Work out the finished part from the listing and answer in its coordinate system (mm). A direction names the side the tool comes from. Coordinates: 2 decimals unless noted, no trailing zeros. Order: outer loops, then holes, each group sorted by start corner. A loop starts at its lowest first (then second) coordinate and runs counter-clockwise, first axis right, second up. Notation, with made-up numbers: M 60,-0.5 L 107,-0.5 A15 ccw 107,19.5 Z; hole C 31.25,-14 d11. An arc over 180 degrees is marked long. Use a Markdown table: item, result. Add a question column.
from build123d import *

# Parameters (mm, degrees)
SKETCH_W        = 3.5
SKETCH_H        = 15
PAD_DEPTH       = 4
SKETCH001_R     = 1.65
PAD001_DEPTH    = 6
POCKET_DEPTH    = 3
POCKET001_DEPTH = 15.001


with BuildPart() as part:
    # Sketch → Pad (new body)
    with BuildSketch(Plane.XY):
        with Locations((1.75, 7.5)):
            Rectangle(SKETCH_W, SKETCH_H)
    extrude(amount=PAD_DEPTH)

    # Sketch001 → Pad001 (join)
    with BuildSketch(Plane.XY):
        with Locations((1.75, 2.5)):
            Circle(SKETCH001_R)
    extrude(amount=PAD001_DEPTH)

    # Sketch002 (on Face1 of Pad001) → Pocket (cut)
    with BuildSketch(Plane.XZ):
        Polygon((3.25, 3.75), (3.25, 0.25), (0.25, 0.25), (0.25, 3.75), (1.75, 3.75), align=None)
    extrude(amount=-POCKET_DEPTH, mode=Mode.SUBTRACT)

    # Sketch003 → Pocket001 (cut, through all)
    with BuildSketch(Plane.XZ):
        Polygon((0.75, 3.75), (1.75, 3.75), (2.75, 3.75), (2.75, 2.25), (0.75, 2.25), align=None)
    extrude(amount=-POCKET001_DEPTH, mode=Mode.SUBTRACT)


solid = part.part
(1) A cutting plane is placed at B-B on x = 1.75. Write down the section's boundary in (y, z).
(2) Straight lines are drawn through the part: line 1 (Z direction, x = 2.1, y = 1.25); line 2 (Z direction, x = 2.1, y = 13); line 3 (X direction, y = 8, z = 2.5). For each, find the intervals that lie inside material, in ascending order.
(3) A cutting plane is placed at A-A on z = 3.2. Write down the section's boundary in (x, y), plus the area to 3 significant figures.
(4) A cutting plane is placed at C-C on y = 11.5. Write down the section's boundary in (x, z), plus the area to 3 significant figures.
(5) Which of the six approach directions +Z, -Z, +X, -X, +Y, -Y give full straight-line access (tool end or side, diameter ignored) to faces 1 (the cylindrical face through (2.64, 3.89, 4.99)), 2 (the flat face through (3.25, 1, 2)), 3 (the flat face through (2.75, 9, 3)), 4 (the flat face through (2, 3, 6)), 5 (the flat face through (2, 15, 2))?
(6) Given P1, Ø1.6, axis at x = 2, y = 7, coming from the +Z side; P2, Ø1.5, axis at x = 1.5, y = 8, coming from the -Z side; P3, Ø1.5, axis at y = 3.5, z = 5.5, coming from the +X side, each flat-ended and moving along its own axis, determine where each tip first touches the part or whether it passes through.
(7) A cutting plane is placed at D-D on z = 1.15. Write down the section's boundary in (x, y).
(8) The mould has two halves that part along Z. Classify faces 6 (the flat face through (2, 9, 2.25)), 7 (the flat face through (2, 9, 4)), 8 (the flat face through (3.5, 7, 2)): pulls with the +Z half, pulls with the -Z half, needs draft (parallel to the pull), parting line crosses it, or undercut.
From the geometry:
| question | item | result |
|---|---|---|
| 1 | outline | M 0,0 L 15,0 L 15,2.25 L 3,2.25 L 3,0.25 L 0,0.25 Z; M 0,3.75 L 15,3.75 L 15,4 L 4.15,4 L 4.15,6 L 0.85,6 L 0.85,4 L 0,4 Z |
| 2 | line 1 | z = 0 to 0.25, 3.75 to 6 |
| 2 | line 2 | z = 0 to 2.25, 3.75 to 4 |
| 2 | line 3 | x = 0 to 0.75, 2.75 to 3.5 |
| 3 | outline | M 0,0 L 0.25,0 L 0.25,3 L 0.75,3 L 0.75,15 L 0,15 Z; M 2.75,3 L 3.25,3 L 3.25,0 L 3.5,0 L 3.5,15 L 2.75,15 Z |
| 3 | area | 19.5 mm2 |
| 4 | outline | M 0,0 L 3.5,0 L 3.5,4 L 0,4 Z; hole M 0.75,2.25 L 2.75,2.25 L 2.75,3.75 L 0.75,3.75 Z |
| 4 | area | 11.0 mm2 |
| 5 | face 1 | +Z |
| 5 | face 2 | -Y |
| 5 | face 3 | +Y, -Y |
| 5 | face 4 | +Z, +X, -X, +Y, -Y |
| 5 | face 5 | +Z, -Z, +X, -X, +Y |
| 6 | P1 | stops at z = 4 |
| 6 | P2 | stops at z = 0 |
| 6 | P3 | stops at x = 3.38 |
| 7 | outline | M 0,0 L 0.25,0 L 0.25,3 L 3.25,3 L 3.25,0 L 3.5,0 L 3.5,15 L 0,15 Z |
| 8 | face 6 | undercut |
| 8 | face 7 | pulls with the +Z half |
| 8 | face 8 | needs draft |
